```python
from build123d import *

# Parameters (mm, degrees)
SKETCH1_W           = 30
SKETCH1_H           = 10
SKETCH1_R           = 1.264247842
BOSS_EXTRUDE1_DEPTH = 5
SKETCH3_R           = 4
BOSS_EXTRUDE2_DEPTH = 4.75
FILLET1_R           = 2
FILLET2_R           = 2
CHAMFER1_SIZE       = 0.8
CUT_EXTRUDE3_REACH  = 34.298
SKETCH6_W           = 3.842122027
SKETCH6_H           = 10
CHAMFER4_START      = 10.25
CHAMFER4_DEPTH      = 9.5
CHAMFER5_SIZE       = 1


with BuildPart() as part:
    # Sketch1 → Boss-Extrude1 (new body)
    with BuildSketch(Plane.XY):
        with Locations((15, 5)):
            Rectangle(SKETCH1_W, SKETCH1_H)
        with Locations((3.444076375, 2.55)):
            Circle(SKETCH1_R, mode=Mode.SUBTRACT)
        with Locations((23.744076375, 2.55)):
            Circle(SKETCH1_R, mode=Mode.SUBTRACT)
    extrude(amount=BOSS_EXTRUDE1_DEPTH)

    # Sketch3 → Boss-Extrude2 (add, symmetric)
    with BuildSketch(Plane.ZY.offset(-15)):
        with Locations((2.568998912, -3.622468738)):
            Circle(SKETCH3_R)
        Polygon((0.404214511, -3.622468738), (1.038265182, -5.153202468), (2.568998912, -5.787253139), (4.099732641, -5.153202468), (4.733783312, -3.622468738), (4.099732641, -2.091735009), (2.568998912, -1.457684338), (1.038265182, -2.091735009), align=None, mode=Mode.SUBTRACT)
    extrude(amount=BOSS_EXTRUDE2_DEPTH, both=True)

    # Fillet1
    # the kernel refuses this fillet: 2 mm, written as the material it adds along each edge
    with BuildSketch(Plane(origin=(19.75, 0, 0.872614451), x_dir=(0, 0, -1), z_dir=(-1, 0, 0))) as fillet1_piece_1:
        with BuildLine():
            CenterArc((2.851261839, -0.291469576), FILLET1_R, 139.283020083, 32.337148469)
            ThreePointArc((1.335379739, 1.013176529), (0.721358104, 0.435852839), (0, 0))
            Line((0, 0), (0.872614451, 0))
        make_face()
    extrude(amount=9.5)
    with BuildSketch(Plane(origin=(19.75, 0, 4.265383373), x_dir=(0, 0, 1), z_dir=(-1, 0, 0))) as fillet1_piece_2:
        with BuildLine():
            CenterArc((2.674069858, 0.488386288), FILLET1_R, 194.13415607, 29.112659272)
            ThreePointArc((1.217251752, -0.881898721), (0.650423795, -0.383257259), (0, 0))
            Line((0, 0), (0.734616627, 0))
        make_face()
    extrude(amount=9.5)

    # Fillet2
    # the kernel refuses this fillet: 2 mm, written as the material it adds along each edge
    with BuildSketch(Plane(origin=(19.75, 0, 0), x_dir=(0, 1, 0), z_dir=(-1, 0, 0))) as fillet2_piece_1:
        with BuildLine():
            CenterArc((0.266521997, 2), FILLET2_R, 229.596597584, 40.403402416)
            Line((-1.029808248, 0.477000363), (-1.159441272, 0.324700399))
            ThreePointArc((-1.159441272, 0.324700399), (-1.143641139, 0.311177078), (-0.029146958, -0.197864739))
            Line((-0.029146958, -0.197864739), (0, -0.2))
            Line((0, -0.2), (0.266521997, -0.2))
            Line((0.266521997, -0.2), (0.266521997, 0))
        make_face()
    extrude(amount=9.5)
    with BuildSketch(Plane(origin=(19.75, 0, 5), x_dir=(0, -0.870596677984774, 0.491997382393317), z_dir=(-1, 0, 0))) as fillet2_piece_2:
        with BuildLine():
            CenterArc((0.615688034, 1.949333304), FILLET2_R, 240.528051524, 42.396189725)
            Line((-0.368306731, 0.208139948), (-0.466706207, 0.034020613))
            Line((-0.466706207, 0.034020613), (-0.098399476, -0.174119336))
            Line((-0.098399476, -0.174119336), (-0.052901843, -0.192876631))
            ThreePointArc((-0.052901843, -0.192876631), (1.052854803, -0.20795909), (1.10774555, -0.19493333))
            Line((1.10774555, -0.19493333), (1.063013048, 0))
        make_face()
    extrude(amount=9.5)

    # Chamfer1
    # the kernel refuses this chamfer: 0.8 mm, written as the material it takes off along each edge
    with BuildSketch(Plane(origin=(19.75, 0.266521997, -2), x_dir=(0, -0.648165122631187, 0.7614998186503384), z_dir=(0, -0.7614998186503384, -0.648165122631187))) as chamfer1_piece_1_section:
        Polygon((2, CHAMFER1_SIZE), (2 + CHAMFER1_SIZE, 0), (2, 0), align=None)
    chamfer1_piece_1 = revolve(axis=Axis((19.75, 0.266521997, -2), (-1, 0, 0)), revolution_arc=99.346805501, mode=Mode.PRIVATE)
    chamfer1_piece_1 = split(chamfer1_piece_1, bisect_by=Plane(origin=(19.75, 0, -2), z_dir=(0, -1, 0)), keep=Keep.TOP, mode=Mode.PRIVATE)
    add(chamfer1_piece_1, mode=Mode.SUBTRACT)
    with BuildSketch(Plane(origin=(19.75, 0.266521997, -2), x_dir=(0, -0.648165122631187, 0.7614998186503384), z_dir=(0, -0.7614998186503384, -0.648165122631187))) as chamfer1_piece_2_section:
        Polygon((2, CHAMFER1_SIZE), (2 + CHAMFER1_SIZE, 0), (2, 0), align=None)
    chamfer1_piece_2 = revolve(axis=Axis((19.75, 0.266521997, -2), (-1, 0, 0)), revolution_arc=99.346805501, mode=Mode.PRIVATE)
    chamfer1_piece_2 = split(chamfer1_piece_2, bisect_by=Plane(origin=(19.75, 0.266521997, 0), z_dir=(0, 0, -1)), keep=Keep.TOP, mode=Mode.PRIVATE)
    add(chamfer1_piece_2, mode=Mode.SUBTRACT)
    with BuildSketch(Plane(origin=(19.75, 0.423050926, 7), x_dir=(0, 0.8566624684959867, -0.515877325602088), z_dir=(0, 0.515877325602088, 0.8566624684959867))) as chamfer1_piece_3_section:
        Polygon((2, CHAMFER1_SIZE), (2 + CHAMFER1_SIZE, 0), (2, 0), align=None)
    chamfer1_piece_3 = revolve(axis=Axis((19.75, 0.423050926, 7), (-1, 0, 0)), revolution_arc=101.340075028, mode=Mode.PRIVATE)
    chamfer1_piece_3 = split(chamfer1_piece_3, bisect_by=Plane(origin=(19.75, 0, 7), z_dir=(0, -1, 0)), keep=Keep.TOP, mode=Mode.PRIVATE)
    add(chamfer1_piece_3, mode=Mode.SUBTRACT)
    with BuildSketch(Plane(origin=(19.75, 0.423050926, 7), x_dir=(0, 0.8566624684959867, -0.515877325602088), z_dir=(0, 0.515877325602088, 0.8566624684959867))) as chamfer1_piece_4_section:
        Polygon((2, CHAMFER1_SIZE), (2 + CHAMFER1_SIZE, 0), (2, 0), align=None)
    chamfer1_piece_4 = revolve(axis=Axis((19.75, 0.423050926, 7), (-1, 0, 0)), revolution_arc=101.340075028, mode=Mode.PRIVATE)
    chamfer1_piece_4 = split(chamfer1_piece_4, bisect_by=Plane(origin=(19.75, 0.423050926, 5), z_dir=(0, 0, 1)), keep=Keep.TOP, mode=Mode.PRIVATE)
    add(chamfer1_piece_4, mode=Mode.SUBTRACT)
    with BuildSketch(Plane(origin=(19.75, -3.622468738, 2.568998912), x_dir=(0, 0.6742532774459821, 0.7385001813495726), z_dir=(0, 0.7385001813495726, -0.6742532774459821))) as chamfer1_piece_5:
        Polygon((4 - CHAMFER1_SIZE, 0), (4, -CHAMFER1_SIZE), (4, 0), align=None)
    revolve(axis=Axis((19.75, -3.622468738, 2.568998912), (1, 0, 0)), revolution_arc=262.799592141, mode=Mode.SUBTRACT)
    with BuildSketch(Plane(origin=(10.25, 0.266521997, -2), x_dir=(0, -0.648165122631187, 0.7614998186503384), z_dir=(0, -0.7614998186503384, -0.648165122631187))) as chamfer1_piece_6_section:
        Polygon((2 + CHAMFER1_SIZE, 0), (2, -CHAMFER1_SIZE), (2, 0), align=None)
    chamfer1_piece_6 = revolve(axis=Axis((10.25, 0.266521997, -2), (-1, 0, 0)), revolution_arc=99.346805501, mode=Mode.PRIVATE)
    chamfer1_piece_6 = split(chamfer1_piece_6, bisect_by=Plane(origin=(10.25, 0, -2), z_dir=(0, -1, 0)), keep=Keep.TOP, mode=Mode.PRIVATE)
    add(chamfer1_piece_6, mode=Mode.SUBTRACT)
    with BuildSketch(Plane(origin=(10.25, 0.266521997, -2), x_dir=(0, -0.648165122631187, 0.7614998186503384), z_dir=(0, -0.7614998186503384, -0.648165122631187))) as chamfer1_piece_7_section:
        Polygon((2 + CHAMFER1_SIZE, 0), (2, -CHAMFER1_SIZE), (2, 0), align=None)
    chamfer1_piece_7 = revolve(axis=Axis((10.25, 0.266521997, -2), (-1, 0, 0)), revolution_arc=99.346805501, mode=Mode.PRIVATE)
    chamfer1_piece_7 = split(chamfer1_piece_7, bisect_by=Plane(origin=(10.25, 0.266521997, 0), z_dir=(0, 0, -1)), keep=Keep.TOP, mode=Mode.PRIVATE)
    add(chamfer1_piece_7, mode=Mode.SUBTRACT)
    with BuildSketch(Plane(origin=(10.25, 0.423050926, 7), x_dir=(0, 0.8566624684959867, -0.515877325602088), z_dir=(0, 0.515877325602088, 0.8566624684959867))) as chamfer1_piece_8_section:
        Polygon((2, -CHAMFER1_SIZE), (2 + CHAMFER1_SIZE, 0), (2, 0), align=None)
    chamfer1_piece_8 = revolve(axis=Axis((10.25, 0.423050926, 7), (-1, 0, 0)), revolution_arc=101.340075028, mode=Mode.PRIVATE)
    chamfer1_piece_8 = split(chamfer1_piece_8, bisect_by=Plane(origin=(10.25, 0, 7), z_dir=(0, -1, 0)), keep=Keep.TOP, mode=Mode.PRIVATE)
    add(chamfer1_piece_8, mode=Mode.SUBTRACT)
    with BuildSketch(Plane(origin=(10.25, 0.423050926, 7), x_dir=(0, 0.8566624684959867, -0.515877325602088), z_dir=(0, 0.515877325602088, 0.8566624684959867))) as chamfer1_piece_9_section:
        Polygon((2, -CHAMFER1_SIZE), (2 + CHAMFER1_SIZE, 0), (2, 0), align=None)
    chamfer1_piece_9 = revolve(axis=Axis((10.25, 0.423050926, 7), (-1, 0, 0)), revolution_arc=101.340075028, mode=Mode.PRIVATE)
    chamfer1_piece_9 = split(chamfer1_piece_9, bisect_by=Plane(origin=(10.25, 0.423050926, 5), z_dir=(0, 0, 1)), keep=Keep.TOP, mode=Mode.PRIVATE)
    add(chamfer1_piece_9, mode=Mode.SUBTRACT)
    with BuildSketch(Plane(origin=(10.25, -3.622468738, 2.568998912), x_dir=(0, 0.6742532774459821, 0.7385001813495726), z_dir=(0, 0.7385001813495726, -0.6742532774459821))) as chamfer1_piece_10:
        Polygon((4 - CHAMFER1_SIZE, 0), (4, CHAMFER1_SIZE), (4, 0), align=None)
    revolve(axis=Axis((10.25, -3.622468738, 2.568998912), (1, 0, 0)), revolution_arc=262.799592141, mode=Mode.SUBTRACT)

    # Cut-Extrude3: up to this face of the body (flat: up to its plane)
    cut_extrude3_end = Plane(part.part.faces().sort_by_distance((30, 5, 2.5))[0])
    # Sketch6 → Cut-Extrude3 (cut, up to the picked face)
    with BuildSketch(Plane(origin=(0, 0, 0), x_dir=(0, 0, -1), z_dir=(1, 0, 0)), mode=Mode.PRIVATE) as cut_extrude3_sk1:
        with Locations((-4.430776166, 5)):
            Rectangle(SKETCH6_W, SKETCH6_H)
    cut_extrude3_tool1 = split(extrude(cut_extrude3_sk1.sketch, amount=CUT_EXTRUDE3_REACH, mode=Mode.PRIVATE), bisect_by=cut_extrude3_end, keep=Keep.BOTH, mode=Mode.PRIVATE)
    add(cut_extrude3_tool1.solids().sort_by(Axis((0, 5, 4.430776), (1, 0, 0)))[0], mode=Mode.SUBTRACT)

    # Chamfer4: read off the stored shape, not the designer's step
    # Chamfer4 outline → Chamfer4 (add)
    with BuildSketch(Plane.YZ.offset(CHAMFER4_START)):
        with BuildLine():
            ThreePointArc((1.304835295, 5.204879857), (0.665907086, 5.014799535), (0, 5.045255026))
            Line((0, 5.045255026), (0, 2.509715152))
            Line((0, 2.509715152), (4, 2.509715152))
            Line((4, 2.509715152), (1.304835295, 5.204879857))
        make_face()
    extrude(amount=CHAMFER4_DEPTH)

    # Chamfer4 2 outline → Chamfer4 2 (revolve, cut)
    with BuildSketch(Plane(origin=(0, 0.423050926, 7), x_dir=(0, 1, 0), z_dir=(0, 0, -1))):
        Polygon((2, 19.75), (2, 18.95), (2.8, 19.75), align=None)
        Polygon((2.8, 10.25), (2, 11.05), (2, 10.25), align=None)
    revolve(axis=Axis((0, 0.423050926, 7), (1, 0, 0)), mode=Mode.SUBTRACT)

    # Chamfer5
    chamfer5_edges = [part.edges().sort_by_distance(p)[0] for p in [
        (19.75, 2, 2.509715152),
        (10.25, 2, 2.509715152),
    ]]
    chamfer(chamfer5_edges, length=CHAMFER5_SIZE)


solid = part.part
```
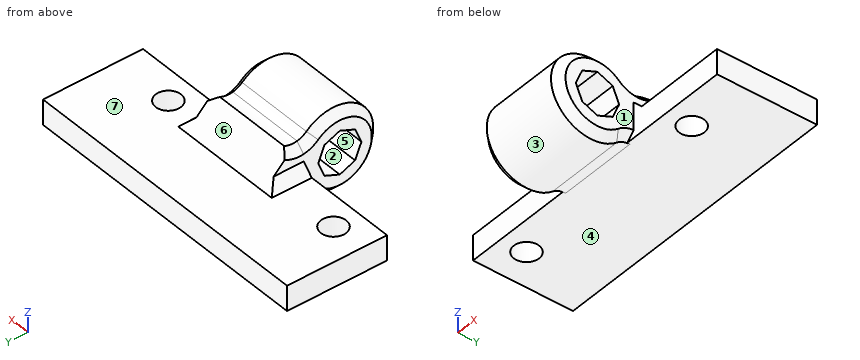
Part model, mm, in its own coordinate system. Face numbers are marked on the shaded views. A direction names the side the tool comes from. Round coordinates to 2 decimals unless told otherwise and drop trailing zeros. Write each loop counter-clockwise with the first axis right and the second up, starting at its lowest first coordinate (ties: lowest second). Pieces come first, ordered by that corner, then holes. Notation, with made-up numbers: M 78.5,-24 L 94.5,-24 A8 cw 94.5,-9 Z; hole C -3.5,1.25 d1. An arc over 180 degrees is marked long. Answer as CSV lines item,"result". Start each with the question number.
1) Band-saw the part on C-C (z = 2). Count the separate pieces of the cut face and the enclosed holes in it, then the cut area to 3 significant figures.
2) Mould opens along Z. For the marked faces 1, 2 and 3 say: +Z half, -Z half, draft (parallel to the pull), parting line (faces both ways), or undercut.
3) Which spindle directions (+Z, -Z, +X, -X, +Y, -Y) get a long thin tool onto all of the face, cutting with end or side? Do the marked faces 4, 5, 6 and 7. Say none if no direction does.
4) Band-saw the part on B-B (x = 17.25). List the corners of the cut face in (y, z).
5) Band-saw the part on A-A (y = 2.55). List the corners of the cut face in (x, z).
6) Drop flat-ended pins along their axis: pin 1 (2 mm diameter, centred on y = -0.5, z = 2, fed in from +X); pin 2 (1.8 mm diameter, centred on x = 23, z = 2, fed in from -Y); pin 3 (1.5 mm diameter, centred on y = -5.5, z = 4, fed in from -X); pin 4 (2 mm diameter, centred on y = -6, z = 5.5, fed in from +X). Give the stop position or say it passes through.
7) Band-saw the part on D-D (x = 8.75). List the corners of the cut face in (y, z), then the cut area to 3 significant figures.
8) Drill centre lines: L1, parallel to X at y = 2.55, z = 0.6; L2, parallel to Z at x = 2, y = 1.5; L3, parallel to Y at x = 17.75, z = 1. Where is each one in solid material? Low to high.
Worked out:
1,separate pieces,"2"
1,enclosed holes,"2"
1,area,"325 mm²"
2,face 1,"draft"
2,face 2,"undercut"
2,face 3,"parting line"
3,face 4,"-Z, +X, -X, +Y"
3,face 5,"+X, -X"
3,face 6,"+Z, +X, -X, +Y"
3,face 7,"+Z, +Y"
4,outline,"M -1.03,-0.48 A2 cw 0.27,0 L 10,0 L 10,2.51 L 4,2.51 L 1.3,5.2 A2 cw -0.93,5.52 A4 ccw long Z; hole M -5.79,2.57 L -5.15,1.04 L -3.62,0.4 L -2.09,1.04 L -1.46,2.57 L -2.09,4.1 L -3.62,4.73 L -5.15,4.1 Z"
5,outline,"M 0,0 L 2.18,0 L 2.18,2.51 L 0,2.51 Z; M 4.71,0 L 22.48,0 L 22.48,2.51 L 20.75,2.51 L 19.75,3.51 L 19.75,3.96 L 10.25,3.96 L 10.25,3.51 L 9.25,2.51 L 4.71,2.51 Z; M 25.01,0 L 30,0 L 30,2.51 L 25.01,2.51 Z"
6,pin 1,"x = 30"
6,pin 2,"y = 0"
6,pin 3,"x = 10.25"
6,pin 4,"x = 19.75"
7,outline,"M 0,0 L 10,0 L 10,2.51 L 0,2.51 Z"
7,area,"25.1 mm²"
8,L1,"0 to 2.18, 4.71 to 22.48, 25.01 to 30"
8,L2,"0 to 2.51"
8,L3,"-7.3 to -5.06, -2.18 to 10"
